Part model, mm, in its own coordinate system. Coordinates: 2 decimals unless noted, no trailing zeros. Order: outer loops, then holes, each group sorted by start corner. A loop starts at its lowest first (then second) coordinate and runs counter-clockwise, first axis right, second up.
Autodesk Inventor part; units mm, degrees
ref_plane "YZ Plane" through (0, 0, 0) normal (1, 0, 0) x (0, 1, 0)
ref_plane "XZ Plane" through (0, 0, 0) normal (0, 1, 0) x (-1, 0, 0)
ref_plane "XY Plane" through (0, 0, 0) normal (0, 0, 1) x (1, 0, 0)
sketch "Esquisse1" plane through (0, 0, 0) normal (1, 0, 0) x (0, 1, 0)
  line L0 (-80, -0.3825) -> (90, -0.3825)
  line L1 (90, -0.3825) -> (155.7273, 23)
  line L2 (155.7273, 23) -> (198, 78)
  line L3 (-80, -0.3825) -> (-102, 18)
  line L4 (-102, 18) -> (-95, 57)
  line L5 (-95, 57) -> (-53, 96)
  line L6 (-53, 96) -> (-9, 96)
  line L7 (-9, 96) -> (60.3686, 39.2438)
  line L8 (60.3686, 39.2438) -> (141.4545, 48)
  line L9 (141.4545, 48) -> (166, 78)
  line L10 (166, 78) -> (198, 78)
  point P0 (0, 0)
  dimension "d0" = 300
  dimension "d1" = 32
  dimension "d2" = 44
  dimension "d3" = 170
extrude "Extrusion1" add sketch "Esquisse1" along normal blind 1.6
fillet "Congé1" radius 50 6 edges at (0.8, -95, 57) (0.8, -80, -0.3825) (0.8, 60.3686, 39.2438) (0.8, 141.4545, 48) (0.8, 155.7273, 23) (0.8, 90, -0.3825)
fillet "Congé2" radius 10 1 edges at (0.8, -102, 18)
fillet "Congé3" radius 10 1 edges at (0.8, 166, 78)
fillet "Congé4" radius 2 1 edges at (0.8, 198, 78)
fillet "Congé5" radius 5 2 edges at (0.8, -9, 96) (0.8, -53, 96)
sketch "Esquisse2" plane through (1.6, 0, 0) normal (1, 0, 0) x (0, 0, -1)
  line L0 (-94.664, -54.4388) -> (-68.3658, -82.7599)
  arc A0 (-23.7165, -100.974) -> (-14.2761, -97.5432) centre (-21.9498, -91.1313) ccw
  line L1 (-14.2761, -97.5432) -> (-11.2486, -93.92)
  line L2 (0.3825, -61.8602) -> (0.3825, 81.3711)
  line L3 (-34.6945, 164.7156) -> (-74.7812, 195.5261)
  line L4 (-78, 193.9403) -> (-78, 170.7388)
  line L5 (-52.5054, 44.1601) -> (-94.8698, -7.6186)
  circle A1 centre (-89.1175, -53.974) radius 2
  circle A2 centre (-19.9498, -95.7558) radius 2
  circle A3 centre (-6.6175, -30.7558) radius 2
  circle A4 centre (-39, 10.1327) radius 2
  circle A5 centre (-20.5549, 80.7442) radius 2
  circle A6 centre (-45.9957, 155.7442) radius 2
  circle A7 centre (-6.6175, 29.2442) radius 2
  circle A8 centre (-74, 189.8806) radius 2
  line L6 (-40.5594, -97.9509) -> (-23.7165, -100.974)
  circle A9 centre (-52.9562, -87.598) radius 2
  circle A10 centre (-89.1175, -8.974) radius 2
  line L7 (-96, -10.7848) -> (-96, -51.0365)
  point P0 (-41.4923, 81.1901)
  point P1 (0, 0)
  dimension "d11" = 4
  dimension "d13" = 4
  dimension "d14" = 4
  dimension "d15" = 4
  dimension "d16" = 4
  dimension "d17" = 4
  dimension "d22" = 2
  dimension "d23" = 5.5
  dimension "d24" = 7
  dimension "d25" = 4
  dimension "d26" = 7
  dimension "d27" = 60
  dimension "d28" = 65
  dimension "d31" = 41.8748
  dimension "d32" = 20.9374
  dimension "d36" = 14
  dimension "d37" = 75
  dimension "d38" = 4
  dimension "d39" = 4
  dimension "d40" = 4
  dimension "d43" = 4
  dimension "d44" = 8
  dimension "d45" = 8
  dimension "d64" = 4
  dimension "d65" = 45
  dimension "d66" = 89.5
  dimension "d67" = 89.5
  dimension "d68" = 47
  dimension "d70" = 32
  dimension "d71" = 57
  dimension "d72" = 51.5
extrude "Extrusion2" cut sketch "Esquisse2" against normal blind 4
sketch "Esquisse3" plane through (1.6, 0, 0) normal (1, 0, 0) x (0, 0, -1)
  line L0 (-34.6945, 164.7156) -> (-74.7812, 195.5261)
  line L1 (-74.3324, 162.9992) -> (-63.8504, 154.423)
  circle A0 centre (-63.2102, 170.4635) radius 5.5
  line L2 (-52.7212, 161.1908) -> (-63.2102, 170.4635)
  line L3 (-63.2102, 170.4635) -> (-73.6991, 179.7361)
  circle A1 centre (-69.2039, 175.7621) radius 1.25
  circle A2 centre (-57.2165, 165.1648) radius 1.25
  point P0 (0, 0)
  dimension "d46" = 11
  dimension "d47" = 12.82
  dimension "d48" = 12.82
  dimension "d50" = 28
  dimension "d51" = 14
  dimension "d52" = 2.5
  dimension "d53" = 2.5
  dimension "d54" = 8
  dimension "d55" = 8
  dimension "d56" = 11.8599
extrude "Extrusion3" cut sketch "Esquisse3" against normal through all
sketch "Esquisse5" plane through (1.6, 0, 0) normal (1, 0, 0) x (0, 0, -1)
  circle A0 centre (-20.5549, 80.7442) radius 2
  line L0 (-52.5054, 44.1601) -> (-94.8698, -7.6186)
  arc A1 (-47.0739, 50.7986) -> (-71.5553, 20.8768) centre (-55.3427, 32.5879) ccw
  line L1 (-47.0739, 50.7986) -> (-71.5553, 20.8768)
  point P0 (-96, -10.7848)
  point P1 (0, 0)
  dimension "d79" = 40
  dimension "d80" = 40
  dimension "d81" = 20
extrude "Extrusion5" add sketch "Esquisse5" against normal blind 1.6 contours L0 A1 L1
fillet "Congé7" radius 20 2 edges at (0.8, 20.8768, 71.5553) (0.8, 51.09, 47.7484)
sketch "Esquisse6" plane through (1.6, 0, 0) normal (1, 0, 0) x (0, 0, -1)
  line L0 (0.3825, -61.8602) -> (0.3825, 81.3711)
  circle A0 centre (-19.9498, -95.7558) radius 2
  circle A1 centre (-64.6175, 39.2442) radius 2
  point P0 (0, 0)
  dimension "d85" = 4
  dimension "d86" = 65
  dimension "d87" = 135
extrude "Extrusion6" cut sketch "Esquisse6" against normal through all contours A1
equation "\"d13\" = d11"
equation "\"d14\" = d11"
equation "\"d15\" = d11"
equation "\"d16\" = d11"
equation "\"d17\" = d11"
equation "\"d25\" = d11"
equation "\"d26\" = d24"
equation "\"d32\" = 0.5 * d31"
equation "\"d38\" = d11"
equation "\"d43\" = d11"
equation "\"d64\" = d11"
equation "\"d67\" = d66"
equation "\"d41\" = d43"
equation "\"d47\" = d48"
equation "\"d51\" = 0.5 * d50"
equation "\"d53\" = d52"
equation "\"d55\" = d54"
properties part number "Cote_Droit" material "Fibre de verre - FR4"
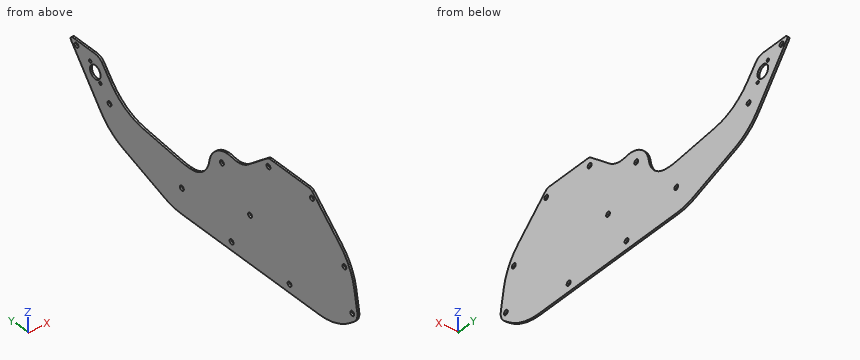
(1) Drop flat-ended pins along their axis: pin 1 (1.5 mm diameter, centred on y = 165.16, z = 57.22, fed in from -X); pin 2 (6.5 mm diameter, centred on y = -87.6, z = 52.96, fed in from -X). Give the stop position or say it passes through.
(2) Slice it at B-B, the plane z = 82. Give the cut face in (x, y), then the cut area to 3 significant figures.
(3) Probe line 1 (Y direction, x = 1.3, z = 69.5); line 2 (Y direction, x = 0.55, z = 62); line 3 (Y direction, x = 1.15, z = 63). List the from-to ranges inside material, lowest first.
(4) Slice it at A-A, the plane x = 0.25. State how many separate pieces and enclosed holes the cut face has, then the cut area to 3 significant figures.
(5) Slice it at C-C, the plane y = 149.5. Give the cut face in (x, z).
Here are the results:
1. pin 1: passes through
1. pin 2: stops at x = 0
2. outline: (0, -68.08) - (1.6, -68.08) - (1.6, 8.11) - (0, 8.11) - close
2. area: 122 mm2
3. line 1: y = -81.54 to 46.71, 159.05 to 174.55, 176.98 to 191.47
3. line 2: y = -88.53 to 51.45, 152.83 to 165.1, 175.83 to 185.7
3. line 3: y = -87.75 to 38.07, 40.42 to 51.06, 153.71 to 164.97, 175.96 to 186.47
4. separate pieces: 1
4. enclosed holes: 14
4. area: 17,200 mm2
5. outline: (0, 21.54) - (1.6, 21.54) - (1.6, 58.64) - (0, 58.64) - close
